Design review of the part built by this model. Coordinates are the model's own, in mm. Round coordinates to 2 decimals unless told otherwise and drop trailing zeros. Order: outer loops, then holes, each group sorted by start corner. A loop starts at its lowest first (then second) coordinate and runs counter-clockwise, first axis right, second up. Notation, with made-up numbers: M 37.5,9 L 67.5,9 A20 cw 67.5,45 Z; hole C 38,54 d6. An arc over 180 degrees is marked long. Write item = value, one per line. Start each with the question number.
```python
from build123d import *

# Parameters (mm, degrees)
BOSS_EXTRUDE1_DEPTH        = 3
M3_5_CLEARANCE_HOLE1_D     = 3.9
M3_5_CLEARANCE_HOLE1_DEPTH = 10
M3_5_CLEARANCE_HOLE1_TIP   = 1.171678207


with BuildPart() as part:
    # Sketch2 → Boss-Extrude1 (new body)
    with BuildSketch(Plane.XY):
        with BuildLine():
            ThreePointArc((-39.28087001, 224.239774099), (-116.578963105, 200.433975785), (-192.012625607, 171.253951952))
            ThreePointArc((-192.012625607, 171.253951952), (-196.936776164, 159.92081589), (-185.905452535, 154.353309203))
            ThreePointArc((-185.905452535, 154.353309203), (-109.656081484, 173.256403098), (-31.987185034, 185.039274932))
            ThreePointArc((-31.987185034, 185.039274932), (-25.021326492, 187.094578874), (-19.248708765, 191.50188464))
            ThreePointArc((-19.248708765, 191.50188464), (-1.783402645, 205.460636468), (19.192242873, 213.200530885))
            ThreePointArc((19.192242873, 213.200530885), (23.830874934, 220.662171124), (16.054107446, 224.750553433))
            ThreePointArc((16.054107446, 224.750553433), (-5.954280946, 220.811707047), (-28.081978855, 224.013059218))
            ThreePointArc((-28.081978855, 224.013059218), (-33.665228727, 224.926425674), (-39.28087001, 224.239774099))
        make_face()
    extrude(amount=-BOSS_EXTRUDE1_DEPTH)

    # M3.5 Clearance Hole1
    with Locations(Plane.XY):
        with Locations((-188.472457343, 162.979460507), (-163.472457343, 173.083498563), (-65.820033869, 203.530407358), (-34.070033869, 204.930522774), (18.040784053, 219.089006289)):
            Hole(M3_5_CLEARANCE_HOLE1_D / 2, depth=M3_5_CLEARANCE_HOLE1_DEPTH)
            with Locations((0, 0, -(M3_5_CLEARANCE_HOLE1_DEPTH + M3_5_CLEARANCE_HOLE1_TIP / 2))):  # 118° drill point
                Cone(0, M3_5_CLEARANCE_HOLE1_D / 2, M3_5_CLEARANCE_HOLE1_TIP, mode=Mode.SUBTRACT)


solid = part.part
```
(1) Consider section A-A, the plane z = -1.1. Write out the cut boundary in (x, y).
(2) Consider section C-C, the plane y = 183. Write out the cut boundary in (x, z).
(3) Draft analysis for pull direction X (two halves, no side actions). For faces 1 (the face through (-2.057, 205.305, -1.479)), 2 (the face through (-115.509, 200.805, -1.479)), 3 (the face through (18.464, 217.185, -1.521)), state which applies: pulls with the +X half, pulls with the -X half, needs draft (parallel to the pull), parting line crosses it, or undercut.
(4) Consider section B-B, the plane x = -83.5. Write out the cut boundary in (y, z), then the cut area to 3 significant figures.
(5) For line 1 along Y through (x, z) = (-187.5, -0.9); line 2 along Y through (x, z) = (-76.5, -1.1); line 3 along Y through (x, z) = (-12, -2.35), list the stretches that pass through material, from the lowest coordinate up. Write a range as [from, to].
Completed:
q1.outline = M -192.01,171.25 A9 ccw -185.91,154.35 A850 cw -31.99,185.04 A20 ccw -19.25,191.5 A70 cw 19.19,213.2 A6 ccw long 16.05,224.75 A70 cw -28.08,224.01 A20 ccw -39.28,224.24 A1150 ccw Z; hole C -188.47,162.98 d3.9; hole C -163.47,173.08 d3.9; hole C -65.82,203.53 d3.9; hole C -34.07,204.93 d3.9; hole C 18.04,219.09 d3.9
q2.outline = M -163.51,-3 L -49.67,-3 L -49.67,0 L -163.51,0 Z
q3.face_1 = pulls with the +X half
q3.face_2 = pulls with the -X half
q3.face_3 = undercut
q4.outline = M 178.05,-3 L 211.35,-3 L 211.35,0 L 178.05,0 Z
q4.area = 99.9 mm2
q5.line_1 = [154.03, 161.29], [164.67, 173.17]
q5.line_2 = [179.19, 213.52]
q5.line_3 = [198.43, 220.97]
